Work out the finished part from the listing and answer in its coordinate system (mm). Face numbers are marked on the shaded views. A direction names the side the tool comes from. Coordinates: 2 decimals unless noted, no trailing zeros. Loops run counter-clockwise (first coordinate to the right, second up) from the corner with the lowest first, then second, coordinate; pieces in that order, holes last. Notation, with made-up numbers: (71.25, 10) -> (127.25, 10) arc R15 ccw to (127.25, 31) -> close; hole circle Ø1 at (74.25, 69). An arc over 180 degrees is marked (long way). Use a Markdown table: item, result.
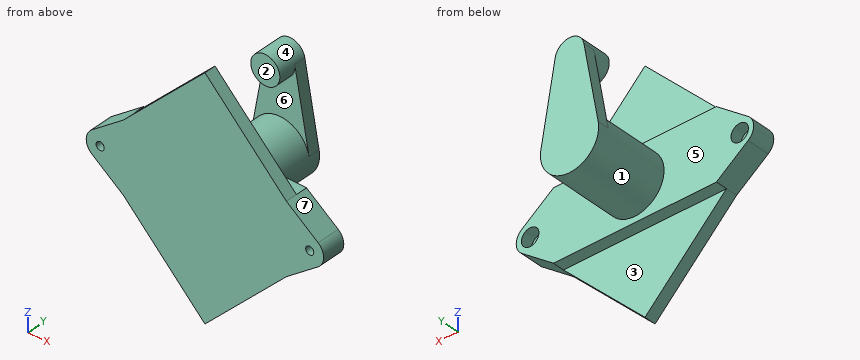
from build123d import *

# Parameters (mm, degrees)
SALIENTE_EXTRUIR1_DEPTH                     = 10
SALIENTE_EXTRUIR1_2_DEPTH                   = 10
CROQUIS2_3_R                                = 25
SALIENTE_EXTRUIR2_DEPTH                     = 20
CROQUIS2_4_R                                = 25
SALIENTE_EXTRUIR3_DEPTH                     = 85
SALIENTE_EXTRUIR4_DEPTH                     = 10
CROQUIS3_3_R                                = 12.5
SALIENTE_EXTRUIR5_DEPTH                     = 25
AVELLANADO_PARA_TORNILLO_CON_CABEZA_2_COUNT = 2
AVELLANADO_PARA_TORNILLO_CON_CABEZA_2_PITCH = 180


with BuildPart() as part:
    # Croquis2 → Saliente-Extruir1 (new body)
    with BuildSketch(Plane(origin=(0, 0, 0), x_dir=(1, 0, 0), z_dir=(0, 1, 0))):
        Polygon((-70, -30), (0, -100), (70, -30), align=None)
    extrude(amount=SALIENTE_EXTRUIR1_DEPTH)



with BuildPart() as body_2:
    # Croquis2 → Saliente-Extruir1 2 (new body)
    with BuildSketch(Plane(origin=(0, 0, 0), x_dir=(1, 0, 0), z_dir=(0, 1, 0))):
        Polygon((0, 100), (70, 30), (-70, 30), align=None)
    extrude(amount=SALIENTE_EXTRUIR1_2_DEPTH)


with BuildPart() as part_1:
    add(part.part)

    add(body_2.part)  # Saliente-Extruir2 merges body 2
    # Croquis2_3 → Saliente-Extruir2 (add)
    with BuildSketch(Plane(origin=(0, 0, 0), x_dir=(1, 0, 0), z_dir=(0, 1, 0))):
        with BuildLine():
            Line((-97.2, 9.6), (-70, 30))
            Line((-70, 30), (70, 30))
            Line((70, 30), (97.2, 9.6))
            ThreePointArc((97.2, 9.6), (102, 0), (97.2, -9.6))
            Line((97.2, -9.6), (70, -30))
            Line((70, -30), (-70, -30))
            Line((-70, -30), (-97.2, -9.6))
            ThreePointArc((-97.2, -9.6), (-102, 0), (-97.2, 9.6))
        make_face()
        Circle(CROQUIS2_3_R, mode=Mode.SUBTRACT)
    extrude(amount=SALIENTE_EXTRUIR2_DEPTH)

    # Croquis2_4 → Saliente-Extruir3 (add)
    with BuildSketch(Plane(origin=(0, 0, 0), x_dir=(1, 0, 0), z_dir=(0, 1, 0))):
        Circle(CROQUIS2_4_R)
    extrude(amount=SALIENTE_EXTRUIR3_DEPTH)

    # Croquis3 → Saliente-Extruir4 (add)
    with BuildSketch(Plane(origin=(0, 85, 0), x_dir=(1, 0, 0), z_dir=(0, 1, 0))):
        with BuildLine():
            ThreePointArc((24.598173775, -4.464285714), (0, -25), (-24.598173775, -4.464285714))
            Line((-24.598173775, -4.464285714), (-12.299086887, -72.232142857))
            ThreePointArc((-12.299086887, -72.232142857), (-1.120583309, -57.550329601), (12.5, -70))
            ThreePointArc((12.5, -70), (12.449670399, -71.120583309), (12.299086887, -72.232142857))
            Line((12.299086887, -72.232142857), (24.598173775, -4.464285714))
        make_face()
    extrude(amount=-SALIENTE_EXTRUIR4_DEPTH)

    # Croquis3_3 → Saliente-Extruir5 (add)
    with BuildSketch(Plane(origin=(0, 85, 0), x_dir=(1, 0, 0), z_dir=(0, 1, 0))):
        with Locations((0, -70)):
            Circle(CROQUIS3_3_R)
    extrude(amount=-SALIENTE_EXTRUIR5_DEPTH)

    # Croquis6 → Avellanado para tornillo con cabeza oval (revolve, cut)
    with BuildSketch(Plane(origin=(90, 20, 0), x_dir=(0, 0, 1), z_dir=(1, 0, 0))):
        Polygon((0, 0), (0, 20), (3.499999985, 20), (3.499999985, 14.60147363), (7.499999986, 10), (7.499999986, 0), align=None)
    avellanado_para_tornillo_con_cabeza_oval = revolve(axis=Axis((90, 26.35, 0), (0, -1, 0)), mode=Mode.SUBTRACT)

    # Avellanado para tornillo con cabeza  2: Avellanado para tornillo con cabeza oval ×2
    with Locations(*[(-i * AVELLANADO_PARA_TORNILLO_CON_CABEZA_2_PITCH, 0, 0) for i in range(1, AVELLANADO_PARA_TORNILLO_CON_CABEZA_2_COUNT)]):
        add(avellanado_para_tornillo_con_cabeza_oval, mode=Mode.SUBTRACT)


solid = part_1.part
Q1. For the marked faces 1, 2 and 3, determine the directions among +Z, -Z, +X, -X, +Y, -Y from which every point of the face is accessible in a straight line to the end or side of a thin tool.
Solved:
| item | result |
|---|---|
| face 1 | none |
| face 2 | +Z, +X, -X |
| face 3 | -Z, +X, -X, +Y |
Q2. Determine the mould class of the marked faces 4, 5, 6 and 7 for opening direction Z: pulls with the +Z half, pulls with the -Z half, needs draft (parallel to the pull), parting line crosses it, or undercut.
Solved:
| item | result |
|---|---|
| face 4 | undercut |
| face 5 | needs draft |
| face 6 | undercut |
| face 7 | pulls with the +Z half |
Q3. Consider line 1 (X direction, y = 17, z = -1); line 2 (Y direction, x = 19, z = -28); line 3 (Y direction, x = 29, z = 44). Determine where each line is inside the solid, lowest interval first. Write a range as [from, to].
Solved:
| item | result |
|---|---|
| line 1 | [-101.96, -97.43], [-82.57, 82.57], [97.43, 101.96] |
| line 2 | [0, 20] |
| line 3 | [0, 10] |
Q4. Section B-B on x = -90 is taken. Determine the outline of the cut face in (y, z), and give its area (3 significant figures).
Solved:
| item | result |
|---|---|
| outline | (0, -15) -> (20, -15) -> (20, -7.5) -> (10, -7.5) -> (5.4, -3.5) -> (0, -3.5) -> close; (0, 3.5) -> (5.4, 3.5) -> (10, 7.5) -> (20, 7.5) -> (20, 15) -> (0, 15) -> close |
| area | 362 mm² |
Q5. Section C-C on x = -58.5 is taken. Determine the outline of the cut face in (y, z).
Solved:
| item | result |
|---|---|
| outline | (0, -41.5) -> (10, -41.5) -> (10, -30) -> (20, -30) -> (20, 30) -> (10, 30) -> (10, 41.5) -> (0, 41.5) -> close |
Q6. Section D-D on y = 57.5 is taken. Determine the outline of the cut face in (x, z).
Solved:
| item | result |
|---|---|
| outline | circle Ø50 at (0, 0) |
Q7. Given pin 1 Ø2 at (x, y) = (-6.5, 54) entering from +Z; pin 2 Ø17 at (x, z) = (90, 0) entering from +Y; pin 3 Ø1 at (x, y) = (15.5, 10) entering from +Z; pin 4 Ø1 at (x, z) = (-32.5, 17) entering from -Y, each flat-ended and moving along its own axis, determine where each tip first touches the part or whether it passes through.
Solved:
| item | result |
|---|---|
| pin 1 | z = 24.39 |
| pin 2 | y = 20 |
| pin 3 | z = 85 |
| pin 4 | y = 0 |
Q8. Section A-A on z = 0 is taken. Determine the outline of the cut face in (x, y).
Solved:
| item | result |
|---|---|
| outline | (-102, 0) -> (-93.5, 0) -> (-93.5, 5.4) -> (-97.5, 10) -> (-97.5, 20) -> (-102, 20) -> close; (-86.5, 0) -> (86.5, 0) -> (86.5, 5.4) -> (82.5, 10) -> (82.5, 20) -> (25, 20) -> (25, 85) -> (-25, 85) -> (-25, 20) -> (-82.5, 20) -> (-82.5, 10) -> (-86.5, 5.4) -> close; (93.5, 0) -> (102, 0) -> (102, 20) -> (97.5, 20) -> (97.5, 10) -> (93.5, 5.4) -> close |
